Verification items for the finished model (mm, model axes). A direction names the side the tool comes from. Round coordinates to 2 decimals unless told otherwise and drop trailing zeros. Order: outer loops, then holes, each group sorted by start corner. A loop starts at its lowest first (then second) coordinate and runs counter-clockwise, first axis right, second up. Notation, with made-up numbers: (1, 84.5) -> (26, 84.5) arc R23 ccw to (26, 109.5) -> close; hole circle Ø4 at (-18, 34.5). An arc over 180 degrees is marked (long way). Answer in a Markdown table with one row per item. Add a question column.
```python
from build123d import *

# Parameters (mm, degrees)
F0_R      = 6
F1_DEPTH  = 4
F2_R      = 6
F2_R_2    = 4.6
F3_DEPTH  = 20
F6_DEPTH  = 25
F8_R      = 4.6
F8_R_2    = 4.35
F9_DEPTH  = 0.3
F10_R     = 0.25
F11_DEPTH = 25
F13_R     = 0.25
F14_DEPTH = 25


with BuildPart() as f1:
    # F0 (on Top) → F1 (new body)
    with BuildSketch(Plane.XY):
        Circle(F0_R)
    extrude(amount=F1_DEPTH)

    # F2 (on face) → F3 (join)
    with BuildSketch(Plane.XY.offset(4)):
        Circle(F2_R)
        Circle(F2_R_2, mode=Mode.SUBTRACT)
    extrude(amount=F3_DEPTH)

    # F5 (on offset) → F6 (cut)
    with BuildSketch(Plane.XZ.offset(10)):
        with BuildLine():
            ThreePointArc((-2.6, 3.75), (-2.8196699141, 4.2803300859), (-3.35, 4.5))
            Line((-3.35, 4.5), (-3.35, 3))
            ThreePointArc((-3.35, 3), (-2.8196699141, 3.2196699141), (-2.6, 3.75))
        make_face()
        with BuildLine():
            Line((3.35, 4.5), (-3.35, 4.5))
            ThreePointArc((-3.35, 4.5), (-2.8196699141, 4.2803300859), (-2.6, 3.75))
            ThreePointArc((-2.6, 3.75), (-2.8196699141, 3.2196699141), (-3.35, 3))
            Line((-3.35, 3), (3.35, 3))
            ThreePointArc((3.35, 3), (2.6, 3.75), (3.35, 4.5))
        make_face()
        with BuildLine():
            Line((-3.35, 3), (-3.35, 4.5))
            ThreePointArc((-3.35, 4.5), (-4.1, 3.75), (-3.35, 3))
        make_face()
        with BuildLine():
            ThreePointArc((4.1, 3.75), (3.8803300859, 4.2803300859), (3.35, 4.5))
            Line((3.35, 4.5), (3.35, 3))
            ThreePointArc((3.35, 3), (3.8803300859, 3.2196699141), (4.1, 3.75))
        make_face()
        with BuildLine():
            Line((3.35, 3), (3.35, 4.5))
            ThreePointArc((3.35, 4.5), (2.6, 3.75), (3.35, 3))
        make_face()
    extrude(amount=-F6_DEPTH, mode=Mode.SUBTRACT)

    # F8 (on offset) → F9 (join)
    with BuildSketch(Plane(origin=(0, 0, 10), x_dir=(1, 0, 0), z_dir=(0, 0, -1))):
        Circle(F8_R)
        Circle(F8_R_2, mode=Mode.SUBTRACT)
    extrude(amount=-F9_DEPTH)

    # F10 (on offset) → F11 (cut)
    with BuildSketch(Plane.XZ.offset(10)):
        with Locations((0, 9.6)):
            Circle(F10_R)
    extrude(amount=-F11_DEPTH, mode=Mode.SUBTRACT)

    # F13 (on offset) → F14 (cut)
    with BuildSketch(Plane.YZ.offset(-15)):
        with Locations((0, 9.6)):
            Circle(F13_R)
    extrude(amount=F14_DEPTH, mode=Mode.SUBTRACT)


solid = f1.part
```
1) Cross-section at D-D, the plane x = -2. Record the boundary of the cut face in (y, z).
2) Cross-section at C-C, the plane z = 9.6. Record the boundary of the cut face in (x, y), and give its area (3 significant figures).
3) Thickness scan on L1, parallel to Z at x = 0, y = 5.2; L2, parallel to Z at x = -2, y = 5.25; L3, parallel to Y at x = 0, z = 10.1. Record the ranges inside material, lowest first. Write a range as [from, to].
4) Cross-section at B-B, the plane x = -0.75. Record the boundary of the cut face in (y, z), and give its area (3 significant figures).
5) Cross-section at A-A, the plane y = 0. Record the boundary of the cut face in (x, z), and give its area (3 significant figures).
6) Depth check by flat-ended pin: P1, Ø3.5, axis at x = 1.5, y = -3, coming from the +Z side; P2, Ø5.5, axis at x = 0, y = 0, coming from the +Z side; P3, Ø4, axis at x = -3.5, z = 12.5, coming from the +Y side; P4, Ø1, axis at y = 4.5, z = 3.5, coming from the +X side. Enter the tip coordinate at first touch or a pass-through.
7) Draft check along Z on faces 5 (the face through (-4.06, -0.07, 3.51)), 6 (the face through (3, -4, 24)), 7 (the face through (2.01, 3.86, 10.15)). Enter one of: +Z half, -Z half, draft (parallel to the pull), parting line (faces both ways), or undercut.
8) Tool access check on faces 1 (the face through (0, 0, 0)), 2 (the face through (0, -5, 4.5)), 3 (the face through (-3.65, -2.8, 17.05)), 4 (the face through (4.25, -1.76, 6.96)). Record the directions out of +Z, -Z, +X, -X, +Y, -Y that give a thin tool (end or side, any length) a straight path to the whole face; none if there is none.
Results below:
| question | item | result |
|---|---|---|
| 1 | outline | (-5.66, 0) -> (5.66, 0) -> (5.66, 3) -> (-5.66, 3) -> close; (-5.66, 4.5) -> (-4.14, 4.5) -> (-4.14, 10) -> (-3.86, 10) -> (-3.86, 10.3) -> (-4.14, 10.3) -> (-4.14, 24) -> (-5.66, 24) -> close; (3.86, 10) -> (4.14, 10) -> (4.14, 4.5) -> (5.66, 4.5) -> (5.66, 24) -> (4.14, 24) -> (4.14, 10.3) -> (3.86, 10.3) -> close |
| 2 | outline | (-5.99, -0.25) arc R6 ccw to (-0.25, -5.99) -> (-0.25, -4.59) arc R4.6 cw to (-4.59, -0.25) -> close; (-5.99, 0.25) -> (-4.59, 0.25) arc R4.6 cw to (-0.25, 4.59) -> (-0.25, 5.99) arc R6 ccw to start; (0.25, -5.99) arc R6 ccw to (5.99, -0.25) -> (4.59, -0.25) arc R4.6 cw to (0.25, -4.59) -> close; (0.25, 4.59) arc R4.6 cw to (4.59, 0.25) -> (5.99, 0.25) arc R6 ccw to (0.25, 5.99) -> close |
| 2 | area | 43.8 mm² |
| 3 | L1 | [0, 3], [4.5, 9.35], [9.85, 24] |
| 3 | L2 | [0, 3], [4.5, 24] |
| 3 | L3 | [-6, -4.35], [4.35, 6] |
| 4 | outline | (-5.95, 0) -> (5.95, 0) -> (5.95, 3) -> (-5.95, 3) -> close; (-5.95, 4.5) -> (-4.54, 4.5) -> (-4.54, 10) -> (-4.28, 10) -> (-4.28, 10.3) -> (-4.54, 10.3) -> (-4.54, 24) -> (-5.95, 24) -> close; (4.28, 10) -> (4.54, 10) -> (4.54, 4.5) -> (5.95, 4.5) -> (5.95, 24) -> (4.54, 24) -> (4.54, 10.3) -> (4.28, 10.3) -> close |
| 4 | area | 91.0 mm² |
| 5 | outline | (-6, 0) -> (6, 0) -> (6, 9.35) -> (4.6, 9.35) -> (4.6, 4) -> (4.06, 4) arc R0.75 cw to (3.35, 3) -> (-3.35, 3) arc R0.75 cw to (-4.06, 4) -> (-4.6, 4) -> (-4.6, 9.35) -> (-6, 9.35) -> close; (-6, 9.85) -> (-4.6, 9.85) -> (-4.6, 10) -> (-4.35, 10) -> (-4.35, 10.3) -> (-4.6, 10.3) -> (-4.6, 24) -> (-6, 24) -> close; (4.35, 10) -> (4.6, 10) -> (4.6, 9.85) -> (6, 9.85) -> (6, 24) -> (4.6, 24) -> (4.6, 10.3) -> (4.35, 10.3) -> close |
| 5 | area | 94.8 mm² |
| 6 | P1 | z = 24 |
| 6 | P2 | z = 3 |
| 6 | P3 | y = 5.81 |
| 6 | P4 | x = 4.47 |
| 7 | face 5 | undercut |
| 7 | face 6 | +Z half |
| 7 | face 7 | draft |
| 8 | face 1 | -Z, +X, -X, +Y, -Y |
| 8 | face 2 | +Y, -Y |
| 8 | face 3 | +Z |
| 8 | face 4 | none |
